Input: part model. Units: mm. Frame: model coordinates. A direction names the side the tool comes from. Give positions to 0.01 mm unless a question says otherwise; leave off trailing zeros. Loops run counter-clockwise (first coordinate to the right, second up) from the corner with the lowest first, then second, coordinate; pieces in that order, holes last. Notation, with made-up numbers: (3, -37) - (31, -37) arc R24 cw to (31, -11) - close; hole circle Ø2 at (-15, 74). An arc over 180 degrees is marked (long way). One line per item, written item: value.
Autodesk Inventor part; units mm, degrees
ref_plane "YZ Plane" through (0, 0, 0) normal (1, 0, 0) x (0, 1, 0)
ref_plane "XZ Plane" through (0, 0, 0) normal (0, 1, 0) x (-1, 0, 0)
ref_plane "XY Plane" through (0, 0, 0) normal (0, 0, 1) x (1, 0, 0)
sketch "Sketch1" plane through (0, 0, 0) normal (0, 0, 1) x (1, 0, 0)
  line L0 (0, 0) -> (0, 50.8)
  line L1 (0, 50.8) -> (76.2, 50.8)
  line L2 (76.2, 50.8) -> (130.0815, 104.6815)
  line L3 (130.0815, 104.6815) -> (166.0026, 68.7605)
  line L4 (166.0026, 68.7605) -> (97.242, 0)
  line L5 (97.242, 0) -> (0, 0)
  circle A0 centre (12.7, 12.7) radius 3.2512
  circle A1 centre (12.7, 38.1) radius 3.2512
  circle A2 centre (38.1, 12.7) radius 3.2512
  circle A3 centre (38.1, 38.1) radius 3.2512
  circle A4 centre (63.5, 12.7) radius 3.2512
  circle A5 centre (63.5, 38.1) radius 3.2512
  circle A6 centre (130.0815, 86.721) radius 3.2512
  circle A7 centre (112.121, 68.7605) radius 3.2512
  circle A8 centre (94.1605, 50.8) radius 3.2512
  circle A9 centre (148.042, 68.7605) radius 3.2512
  circle A10 centre (130.0815, 50.8) radius 3.2512
  circle A11 centre (112.121, 32.8395) radius 3.2512
  dimension "d0" = 50.8
  dimension "d1" = 76.2
  dimension "d2" = 76.2
  dimension "d3" = 135
  dimension "d4" = 50.8
  dimension "d5" = 6.5024
  dimension "d6" = 12.7
  dimension "d7" = 12.7
  dimension "d10" = 25.4
  dimension "d13" = 25.4
  dimension "d16" = 6.5024
  dimension "d17" = 12.7
  dimension "d18" = 12.7
  dimension "d21" = 25.4
  dimension "d24" = 25.4
extrude "Extrusion1" add sketch "Sketch1" along normal blind 6.35
properties part number "2x3 Vplate"
Item 1: Section D-D, the plane y = 38.1. Output: boundary loops of the cut face in (x, z), and give its area (3 significant figures).
Verdict:
outline: (0, 0) - (9.45, 0) - (9.45, 6.35) - (0, 6.35) - close; (15.95, 0) - (34.85, 0) - (34.85, 6.35) - (15.95, 6.35) - close; (41.35, 0) - (60.25, 0) - (60.25, 6.35) - (41.35, 6.35) - close; (66.75, 0) - (135.34, 0) - (135.34, 6.35) - (66.75, 6.35) - close
area: 736 mm^2
Item 2: Material intervals for L1, parallel to Y at x = 12.7, z = 3.25; L2, parallel to Y at x = 41, z = 2.25; L3, parallel to X at y = 48, z = 3, sorted ascending.
Verdict:
L1: y = 0 to 9.45, 15.95 to 34.85, 41.35 to 50.8
L2: y = 0 to 11.23, 14.17 to 36.63, 39.57 to 50.8
L3: x = 0 to 92.51, 95.81 to 128.43, 131.73 to 145.24
Item 3: Access query for faces 1 (the face through (82, 41, 6.35)), 2 (the face through (38, 50.8, 3)). Directions: +Z, -Z, +X, -X, +Y, -Y. A direction counts if a zero-diameter tool reaches every point of the face in a straight line with its end or side. Return the directions, or none.
Verdict:
face 1: +Z, +X, -X, +Y, -Y
face 2: +Z, -Z, -X, +Y
Item 4: Section C-C, the plane z = 1. Count the separate pieces of the cut face and the enclosed holes in it, and give its area (3 significant figures).
Verdict:
separate pieces: 1
enclosed holes: 12
area: 8,410 mm^2
Item 5: Section A-A, the plane x = 38.1. Output: boundary loops of the cut face in (y, z), and give its area (3 significant figures).
Verdict:
outline: (0, 0) - (9.45, 0) - (9.45, 6.35) - (0, 6.35) - close; (15.95, 0) - (34.85, 0) - (34.85, 6.35) - (15.95, 6.35) - close; (41.35, 0) - (50.8, 0) - (50.8, 6.35) - (41.35, 6.35) - close
area: 240 mm^2
Item 6: Pin query (flat end, axial travel): P1, Ø3, axis at x = 69.5, z = 3, coming from the +Y side; P2, Ø10.5, axis at x = 38.1, y = 12.7, coming from the -Z side; P3, Ø3, axis at x = 91.5, z = 3, coming from the +Y side. Return the tip coordinate at first contact, or that it passes through.
Verdict:
P1: stops at y = 50.8
P2: stops at z = 0
P3: stops at y = 67.6
Item 7: Section B-B, the plane y = 12.7. Output: boundary loops of the cut face in (x, z), and give its area (3 significant figures).
Verdict:
outline: (0, 0) - (9.45, 0) - (9.45, 6.35) - (0, 6.35) - close; (15.95, 0) - (34.85, 0) - (34.85, 6.35) - (15.95, 6.35) - close; (41.35, 0) - (60.25, 0) - (60.25, 6.35) - (41.35, 6.35) - close; (66.75, 0) - (109.94, 0) - (109.94, 6.35) - (66.75, 6.35) - close
area: 574 mm^2
Item 8: Draft query along Y for faces 3 (the face through (9.45, 12.56, 3.13)), 4 (the face through (82, 41, 0)), 5 (the face through (147.791, 86.972, 3.131)), 6 (the face through (108.873, 32.697, 3.131)). Return one class per face: pulls with the +Y half, pulls with the -Y half, needs draft (parallel to the pull), parting line crosses it, or undercut.
Verdict:
face 3: undercut
face 4: needs draft
face 5: pulls with the +Y half
face 6: undercut
